```python
from build123d import *

# Parameters (mm, degrees)
F1_DEPTH = 12.7
F2_R     = 25.4
F4_DEPTH = 254
F5_R     = 50.8
F6_R     = 2.15265
F7_DEPTH = 12.7


with BuildPart() as f1:
    # F0 (on Top) → F1 (new body)
    with BuildSketch(Plane.XY):
        with BuildLine():
            Line((-254, -635), (0, -635))
            Line((0, -635), (0, 0))
            ThreePointArc((0, 0), (-33.5193668575, 141.9903165712), (-127, 254))
            ThreePointArc((-127, 254), (-220.4806331425, 141.9903165712), (-254, 0))
            Line((-254, 0), (-254, -635))
        make_face()
    extrude(amount=F1_DEPTH)

    # F2
    f2_edges = [f1.edges().sort_by_distance(p)[0] for p in [
        (-127, 254, 6.35),
    ]]
    fillet(f2_edges, radius=F2_R)

    # F3 (on face) → F4 (join, through all)
    with BuildSketch(Plane(origin=(-254, 0, 0), x_dir=(0, -1, 0), z_dir=(-1, 0, 0))):
        with BuildLine():
            ThreePointArc((658.0090131096, 15.7291940429), (646.6037784884, 13.4605518239), (635, 12.7))
            Line((635, 12.7), (635, 0))
            ThreePointArc((635, 0), (648.2614611296, 0.8692020844), (661.2960149824, 3.461936049))
            Line((661.2960149824, 3.461936049), (759.4340789334, 29.7579510314))
            Line((759.4340789334, 29.7579510314), (756.1470770606, 42.0252090253))
            Line((756.1470770606, 42.0252090253), (658.0090131096, 15.7291940429))
        make_face()
    extrude(amount=-F4_DEPTH)

    # F5
    f5_edges = [f1.edges().sort_by_distance(p)[0] for p in [
        (0, -757.790578, 35.89158),
        (-254, -757.790578, 35.89158),
    ]]
    fillet(f5_edges, radius=F5_R)

    # F6 (on face) → F7 (cut, through all)
    with BuildSketch(Plane.XY.offset(12.7)):
        with Locations((-127, -520.7)):
            Circle(F6_R)
        with Locations((-127, -622.3)):
            Circle(F6_R)
        with Locations((-241.3, -12.7)):
            Circle(F6_R)
        with Locations((-12.7, -12.7)):
            Circle(F6_R)
    extrude(amount=-F7_DEPTH, mode=Mode.SUBTRACT)


solid = f1.part
```
Geometry check sheet. Reference: the model listing, model coordinates, mm. A direction names the side the tool comes from. Coordinates: 2 decimals unless noted, no trailing zeros. Write each loop counter-clockwise with the first axis right and the second up, starting at its lowest first coordinate (ties: lowest second). Pieces come first, ordered by that corner, then holes. Notation, with made-up numbers: M 6.25,68 L 38.25,68 A12 cw 38.25,74 Z; hole C -32.75,-0.5 d3. An arc over 180 degrees is marked long. One line per item, written item: value. Start each with the question number.
(1) Scan lines: line 1 along X through (y, z) = (-520.7, 5); line 2 along X through (y, z) = (-520, 4); line 3 along Z through (x, y) = (-198, 159.5). Record each from-to range of solid material in increasing order. Write a range as [from, to].
(2) Depth check by flat-ended pin: pin 1 (1.5 mm diameter, centred on y = -135, z = 10.5, fed in from +X); pin 2 (4 mm diameter, centred on x = -29, y = -340, fed in from +Z). Enter the tip coordinate at first touch or a pass-through.
(3) Sectioned sample at C-C, the plane y = 186. Enter the section's corners in (x, z), and give its area (3 significant figures).
(4) Sectioned sample at A-A, the plane y = -80. Enter the section's corners in (x, z).
(5) Sectioned sample at B-B, the plane x = -95. Enter the section's corners in (y, z).
(6) Tool access check on faces 1 (the face through (-129, -188, 12.7)), 2 (the face through (-254, -350, 8)). Record the directions out of +Z, -Z, +X, -X, +Y, -Y that give a thin tool (end or side, any length) a straight path to the whole face; none if there is none.
Filled sheet:
1. line 1: [-254, -129.15], [-124.85, 0]
1. line 2: [-254, -129.04], [-124.96, 0]
1. line 3: [0, 12.7]
2. pin 1: x = 0
2. pin 2: z = 12.7
3. outline: M -193.81,0 L -60.19,0 L -60.19,12.7 L -193.81,12.7 Z
3. area: 1,700 mm²
4. outline: M -254,0 L 0,0 L 0,12.7 L -254,12.7 Z
5. outline: M -759.43,29.76 L -661.3,3.46 A101.6 ccw -635,0 L 226.5,0 L 226.5,12.7 L -635,12.7 A88.9 cw -658.01,15.73 L -756.15,42.03 Z
6. face 1: +Z, +X, -X, +Y
6. face 2: +Z, -Z, -X, +Y, -Y
